from build123d import *

# Parameters (mm, degrees)
SKETCH4_R           = 5.3578125
BOSS_EXTRUDE2_DEPTH = 6.35
CUT_EXTRUDE1_DEPTH  = 1277.826258948
FILLET1_R           = 2.54


with BuildPart() as part:
    # Sketch4 → Boss-Extrude2 (new body)
    # profile 1 of 2: a face of its own
    with BuildSketch(Plane(origin=(0, 0, 0), x_dir=(1, 0, 0), z_dir=(0, 1, 0))):
        Polygon((234.979236566, 1078.971634327), (-356.170330123, 0), (682.689669877, 0), (429.674039163, 609.761730508), (381.000338514, 727.064206463), align=None)
        with Locations(Location((-178.370330123, 38.1, 0), (0, 0, 270))):
            Circle(SKETCH4_R, mode=Mode.SUBTRACT)
        with Locations(Location((-259.300975608, 137.16, 0), (0, 0, 270))):
            Circle(SKETCH4_R, mode=Mode.SUBTRACT)
        with Locations(Location((-93.289784566, 440.165155055, 0), (0, 0, 270))):
            Circle(SKETCH4_R, mode=Mode.SUBTRACT)
        with Locations(Location((504.889669877, 38.1, 0), (0, 0, 270))):
            Circle(SKETCH4_R, mode=Mode.SUBTRACT)
        with Locations(Location((489.29326545, 416.375307605, 0), (0, 0, 270))):
            Circle(SKETCH4_R, mode=Mode.SUBTRACT)
        with Locations(Location((61.094542054, 721.948850069, 0), (0, 0, 270))):
            Circle(SKETCH4_R, mode=Mode.SUBTRACT)
        with Locations(Location((303.667495105, 863.729056592, 0), (0, 0, 270))):
            Circle(SKETCH4_R, mode=Mode.SUBTRACT)
        with Locations(Location((201.97392089, 979.083189991, 0), (0, 0, 270))):
            Circle(SKETCH4_R, mode=Mode.SUBTRACT)
    # profile 2 of 2: a face of its own
    with BuildSketch(Plane(origin=(0, 0, 0), x_dir=(1, 0, 0), z_dir=(0, 1, 0))):
        Polygon((429.674039163, 609.761730508), (381.000338514, 727.064206463), (398.595709907, 734.36526156), (447.269410556, 617.062785606), align=None)
    extrude(amount=BOSS_EXTRUDE2_DEPTH)

    # Sketch5 → Cut-Extrude1 (cut, through all)
    with BuildSketch(Plane(origin=(0, 6.35, 0), x_dir=(1, 0, 0), z_dir=(0, 1, 0))):
        with BuildLine():
            Line((-250.361653335, 116.472417753), (-238.157149202, 138.748191115))
            ThreePointArc((-238.157149202, 138.748191115), (-220.917010455, 143.783825729), (-215.88137584, 126.543686982))
            Line((-215.88137584, 126.543686982), (-228.085879973, 104.26791362))
            ThreePointArc((-228.085879973, 104.26791362), (-245.326018721, 99.232279006), (-250.361653335, 116.472417753))
        make_face()
        with BuildLine():
            Line((-191.070330123, 81.28), (-165.670330123, 81.28))
            ThreePointArc((-165.670330123, 81.28), (-152.970330123, 68.58), (-165.670330123, 55.88))
            Line((-165.670330123, 55.88), (-191.070330123, 55.88))
            ThreePointArc((-191.070330123, 55.88), (-203.770330123, 68.58), (-191.070330123, 81.28))
        make_face()
        with BuildLine():
            Line((-83.493702347, 421.041338954), (-71.289198214, 443.317112316))
            ThreePointArc((-71.289198214, 443.317112316), (-54.049059466, 448.35274693), (-49.013424852, 431.112608183))
            Line((-49.013424852, 431.112608183), (-61.217928985, 408.836834821))
            ThreePointArc((-61.217928985, 408.836834821), (-78.458067732, 403.801200206), (-83.493702347, 421.041338954))
        make_face()
        with BuildLine():
            Line((211.607161604, 959.662154075), (223.811665737, 981.937927436))
            ThreePointArc((223.811665737, 981.937927436), (241.051804485, 986.973562051), (246.087439099, 969.733423303))
            Line((246.087439099, 969.733423303), (233.882934966, 947.457649942))
            ThreePointArc((233.882934966, 947.457649942), (216.642796219, 942.422015327), (211.607161604, 959.662154075))
        make_face()
        with BuildLine():
            Line((70.0689996, 701.325397046), (82.328936684, 723.702347141))
            ThreePointArc((82.328936684, 723.702347141), (99.569075432, 728.737981755), (104.604710046, 711.497843008))
            Line((104.604710046, 711.497843008), (92.344772962, 689.120892913))
            ThreePointArc((92.344772962, 689.120892913), (75.104634214, 684.085258298), (70.0689996, 701.325397046))
        make_face()
        with BuildLine():
            Line((467.764558528, 421.867197937), (477.499298658, 398.406702746))
            ThreePointArc((477.499298658, 398.406702746), (470.636421128, 381.809085085), (454.038803467, 388.671962616))
            Line((454.038803467, 388.671962616), (444.304063337, 412.132457807))
            ThreePointArc((444.304063337, 412.132457807), (451.166940868, 428.730075467), (467.764558528, 421.867197937))
        make_face()
        with BuildLine():
            Line((492.961263737, 81.28), (518.361263737, 81.28))
            ThreePointArc((518.361263737, 81.28), (531.061263737, 68.58), (518.361263737, 55.88))
            Line((518.361263737, 55.88), (492.961263737, 55.88))
            ThreePointArc((492.961263737, 55.88), (480.261263737, 68.58), (492.961263737, 81.28))
        make_face()
        with BuildLine():
            Line((282.363160209, 868.680215609), (292.097900339, 845.219720419))
            ThreePointArc((292.097900339, 845.219720419), (285.235022808, 828.622102758), (268.637405148, 835.484980289))
            Line((268.637405148, 835.484980289), (258.902665018, 858.94547548))
            ThreePointArc((258.902665018, 858.94547548), (265.765542549, 875.54309314), (282.363160209, 868.680215609))
        make_face()
    extrude(amount=-CUT_EXTRUDE1_DEPTH, mode=Mode.SUBTRACT)

    # Fillet1
    fillet1_edges = [part.edges().sort_by_distance(p)[0] for p in [
        (682.689669877, 3.175, 0),
        (-356.170330123, 3.175, 0),
        (234.979236566, 3.175, -1078.971634327),
        (381.000338514, 3.175, -727.064206463),
        (429.674039163, 3.175, -609.761730508),
        (447.269410556, 3.175, -617.062785606),
        (398.595709907, 3.175, -734.36526156),
    ]]
    fillet(fillet1_edges, radius=FILLET1_R)


solid = part.part
For this review, take the finished solid that the model builds, in its own axes (mm). Round coordinates to 2 decimals unless told otherwise and drop trailing zeros. Order: outer loops, then holes, each group sorted by start corner. A loop starts at its lowest first (then second) coordinate and runs counter-clockwise, first axis right, second up. Notation, with made-up numbers: M -17.75,47.5 L 36.25,47.5 A17 cw 36.25,63.5 Z; hole C 24,57.5 d8. An arc over 180 degrees is marked long. Use a Markdown table: item, result. Add a question column.
Item 1: To check wall thickness, follow line 1 along X through (y, z) = (4.5, -137.16); line 2 along Z through (x, y) = (124, 2.5); line 3 along Z through (x, y) = (217, 5). State the ranges of each line that lie inside material, in increasing order.
Item 2: Add section C-C, the plane y = 5.25. State how many separate pieces and enclosed holes the cut face has, then the cut area to 3 significant figures.
Item 3: Add section D-D, the plane x = 344.5. Give the boundary of the cut face in (y, z).
Item 4: Add section B-B, the plane z = -908. Give the boundary of the cut face in (x, y), then the cut area to 3 significant figures.
Item 5: Add section A-A, the plane z = -68.58. Give the boundary of the cut face in (x, y), then the cut area to 3 significant figures.
Item 6: Insertion check: pin 1 (8.5 mm diameter, centred on x = 489.29, z = -416.38, fed in from -Y); pin 2 (3 mm diameter, centred on x = 492, y = 2.5, fed in from -Z); pin 3 (1.5 mm diameter, centred on y = 1, z = -300, fed in from -X); pin 4 (1.9 mm diameter, centred on x = -181.5, y = 4, fed in from -Z). Each pin has a flat end and moves straight along its axis. Give the tip position at first contact, or say it passes through.
Geometry results:
| question | item | result |
|---|---|---|
| 1 | line 1 | x = -281.02 to -264.66, -253.94 to -239.03, -215.15 to 625.78 |
| 1 | line 2 | z = -876.41 to 0 |
| 1 | line 3 | z = -1046.16 to -969.51, -942.23 to 0 |
| 2 | separate pieces | 1 |
| 2 | enclosed holes | 16 |
| 2 | area | 553,000 mm² |
| 3 | outline | M 0,-815.03 L 6.35,-815.03 L 6.35,0 L 0,0 Z |
| 4 | outline | M 141.31,0 L 305.92,0 L 305.92,6.35 L 141.31,6.35 Z |
| 4 | area | 1,050 mm² |
| 5 | outline | M -318.6,0 L -203.77,0 L -203.77,6.35 L -318.6,6.35 Z; M -152.97,0 L 480.26,0 L 480.26,6.35 L -152.97,6.35 Z; M 531.06,0 L 654.23,0 L 654.23,6.35 L 531.06,6.35 Z |
| 5 | area | 5,530 mm² |
| 6 | pin 1 | passes through |
| 6 | pin 2 | stops at z = -463.17 |
| 6 | pin 3 | stops at x = -192.22 |
| 6 | pin 4 | stops at z = -320.54 |
